Source: CAD feature listing. Evaluate the final solid. Frame: model axes, mm. A direction names the side the tool comes from. Coordinates: 2 decimals unless noted, no trailing zeros. Order: outer loops, then holes, each group sorted by start corner. A loop starts at its lowest first (then second) coordinate and runs counter-clockwise, first axis right, second up.
```python
from build123d import *

# Parameters (mm, degrees)
F1_DEPTH = 17.78
F2_R     = 6.35
F3_DEPTH = 25.4


with BuildPart() as f1:
    # F0 (on Top) → F1 (new body)
    with BuildSketch(Plane.XY):
        with BuildLine():
            Line((133.935379, 42.337351), (-170.864621, 42.337351))
            ThreePointArc((-170.864621, 42.337351), (-183.564621, 29.637351), (-170.864621, 16.937351))
            Line((-170.864621, 16.937351), (133.935379, 16.937351))
            ThreePointArc((133.935379, 16.937351), (146.635379, 29.637351), (133.935379, 42.337351))
        make_face()
    extrude(amount=F1_DEPTH)

    # F2 (on face) → F3 (join)
    with BuildSketch(Plane.XY.offset(17.78)):
        with Locations((133.935379, 29.637351)):
            Circle(F2_R)
        with Locations((-170.864621, 29.637351)):
            Circle(F2_R)
    extrude(amount=F3_DEPTH)


solid = f1.part
```
Q1. Pin query (flat end, axial travel): P1, Ø12, axis at x = -119, z = 29, coming from the +Y side; P2, Ø10, axis at y = 38.5, z = 8.5, coming from the +X side; P3, Ø10, axis at y = 39, z = 17, coming from the -X side; P4, Ø12.5, axis at x = -91.5, y = 24.5, coming from the +Z side. Return the tip coordinate at first contact, or that it passes through.
Solutions:
P1: passes through
P2: stops at x = 146.03
P3: stops at x = -182.79
P4: stops at z = 17.78
Q2. Set-up query: faces 1 (the flat face through (-16, 42.337, 9)), 2 (the cylindrical face through (-172.24, 23.44, 30.3)). Return all of +Z, -Z, +X, -X, +Y, -Y with unobstructed straight access to the full face (end or side cutting, diameter ignored); none if empty.
Solutions:
face 1: +Z, -Z, +X, -X, +Y
face 2: +Z
Q3. Section query B-B on z = 30.5. Output: boundary loops of the cut face in (x, y).
Solutions:
outline: circle Ø12.7 at (-170.86, 29.64); circle Ø12.7 at (133.94, 29.64)
Q4. Material intervals for line 1 along X through (y, z) = (30.5, 24); line 2 along Z through (x, y) = (69.5, 28.75); line 3 along X through (y, z) = (34, 40), sorted ascending.
Solutions:
line 1: x = -177.16 to -164.57, 127.64 to 140.23
line 2: z = 0 to 17.78
line 3: x = -175.48 to -166.25, 129.32 to 138.55
Q5. Section query D-D on z = 14. Output: boundary loops of the cut face in (x, y).
Solutions:
outline: (-170.86, 16.94) - (133.94, 16.94) arc R12.7 ccw to (133.94, 42.34) - (-170.86, 42.34) arc R12.7 ccw to start
Q6. Section query C-C on x = -61. Output: boundary loops of the cut face in (y, z).
Solutions:
outline: (16.94, 0) - (42.34, 0) - (42.34, 17.78) - (16.94, 17.78) - close
Q7. Section query A-A on y = 26.75. Output: boundary loops of the cut face in (x, z).
Solutions:
outline: (-183.23, 0) - (146.3, 0) - (146.3, 17.78) - (139.59, 17.78) - (139.59, 43.18) - (128.28, 43.18) - (128.28, 17.78) - (-165.21, 17.78) - (-165.21, 43.18) - (-176.52, 43.18) - (-176.52, 17.78) - (-183.23, 17.78) - close
